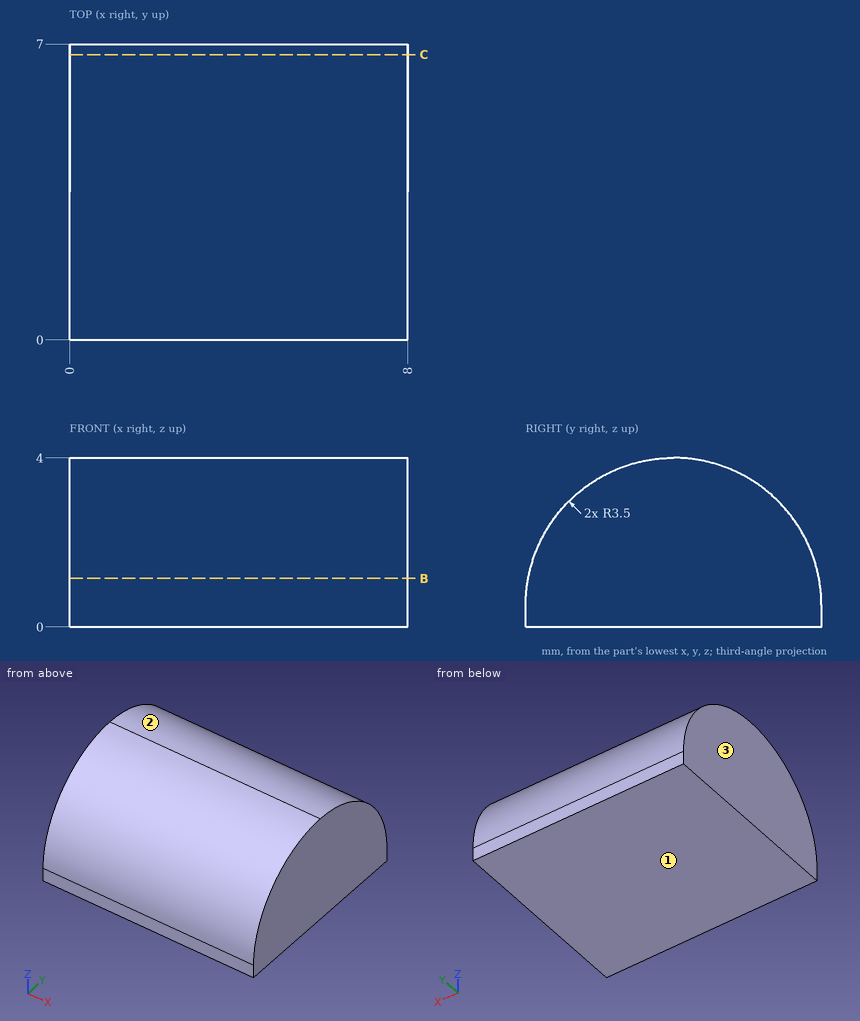
Design review of the part shown in the three views and the two pictorial views. Dimensions are in mm from the part's minimum x, y and z. Round coordinates to 2 decimals unless told otherwise and drop trailing zeros. Loops run counter-clockwise (first coordinate to the right, second up) from the corner with the lowest first, then second, coordinate; pieces in that order, holes last.
1) Consider section C-C on y = 6.75. State the section outline as (x, z) points.
Values follow:
outline: (0, 0) - (8, 0) - (8, 1.8) - (0, 1.8) - close
2) The part is to be moulded in two halves that separate along Z. For the marked faces 1, 2 and 3, say which applies: pulls with the +Z half, pulls with the -Z half, needs draft (parallel to the pull), parting line crosses it, or undercut.
Values follow:
face 1: pulls with the -Z half
face 2: pulls with the +Z half
face 3: needs draft
3) Consider section B-B on z = 1.15. State the section outline as (x, y) points, then the cut area to 3 significant figures.
Values follow:
outline: (0, 0.06) - (8, 0.06) - (8, 6.94) - (0, 6.94) - close
area: 55.0 mm2
4) Wall thickness on line 1 along Y through (x, z) = (3, 1.25); line 2 along Z through (x, y) = (7.5, 0.75) (1 decimal); line 3 along Z through (x, y) = (7, 1.25): over which ranges is each line inside the solid? List them lowest first.
Values follow:
line 1: y = 0.08 to 6.92
line 2: z = 0 to 2.7
line 3: z = 0 to 3.18
